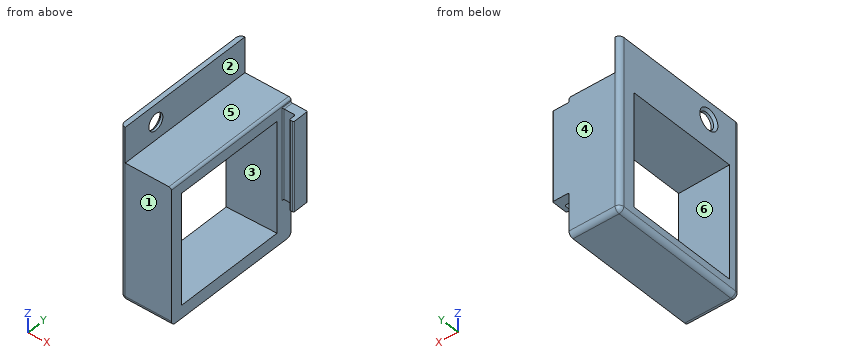
Autodesk Inventor part; units mm, degrees
ref_plane "YZ Plane" through (0, 0, 0) normal (1, 0, 0) x (0, 1, 0)
ref_plane "XZ Plane" through (0, 0, 0) normal (0, 1, 0) x (-1, 0, 0)
ref_plane "XY Plane" through (0, 0, 0) normal (0, 0, 1) x (1, 0, 0)
sketch "Boceto1" plane through (0, 0, 0) normal (1, 0, 0) x (0, 1, 0)
  line L0 (0, 0) -> (-47.8, 0)
  line L1 (-47.8, 0) -> (-47.8, 48)
  line L2 (-47.8, 48) -> (0, 48)
  line L3 (0, 48) -> (0, 0)
  line L4 (-23.9, 48) -> (-23.9, 53)
  line L5 (-23.9, 0) -> (-23.9, -5)
  line L6 (0, 24) -> (5, 24)
  line L7 (-47.8, 24) -> (-52.8, 24)
  line L8 (5, -5) -> (-52.8, -5)
  line L9 (-52.8, -5) -> (-52.8, 53)
  line L10 (-52.8, 53) -> (5, 53)
  line L11 (5, 53) -> (5, -5)
  dimension "d0" = 47.8
  dimension "d1" = 48
  dimension "d2" = 5
  dimension "d3" = 5
  dimension "d4" = 5
  dimension "d5" = 5
extrude "Extrusión1" add sketch "Boceto1" along normal blind 21.5 contours L3 L6 L11 L8 L5 L0 | L5 L8 L9 L7 L1 L0 | L3 L2 L4 L10 L11 L6 | L7 L9 L10 L4 L2 L1
sketch "Boceto2" plane through (0, 0, 0) normal (-1, 0, 0) x (0, 0, 1)
  line L0 (53, 5) -> (53, -52.8)
  line L1 (53, 5) -> (68, 5)
  line L2 (68, 5) -> (68, -52.8)
  line L3 (68, -52.8) -> (53, -52.8)
  line L4 (53, -52.8) -> (53, 5)
  point P0 (0, 0)
  dimension "d8" = 15
extrude "Extrusión2" add sketch "Boceto2" against normal blind 2
sketch "Boceto3" plane through (21.5, 0, 0) normal (1, 0, 0) x (0, 0, -1)
  line L0 (-51, 5) -> (-13, 5)
  line L1 (-13, 3) -> (-51, 3)
  line L2 (-51, 5) -> (-51, 3)
  line L3 (-13, 5) -> (-13, 3)
extrude "Extrusión3" add sketch "Boceto3" along normal blind 7
sketch "Boceto4" plane through (21.5, 3, 13) normal (0, -1, 0) x (1, 0, 0)
  line L0 (0, 38) -> (7, 38)
  line L1 (0, 0) -> (7, 0)
  line L2 (7, 38) -> (5.2, 38)
  line L3 (5.2, 38) -> (5.2, 0)
  line L4 (5.2, 0) -> (7, 0)
  line L5 (7, 0) -> (7, 38)
  point P0 (-21.5, -13)
  point P1 (7, 0)
  dimension "d16" = 1.8
extrude "Extrusión4" add sketch "Boceto4" along normal blind 3
sketch "Boceto5" plane through (0, 0, 0) normal (-1, 0, 0) x (0, 0, 1)
  line L0 (60.5, 5) -> (60.5, -37.5)
  dimension "d19" = 42.5
hole "Agujero1" at (0, -37.5, 60.5) direction (1, 0, 0) diameter 7 depth 2 countersink diameter 9 countersink angle 90
fillet "Empalme3" radius 0.5 2 edges at (28.5, 0, 32) (26.7, 0, 32)
sketch "Boceto6" plane through (21.5, 0, 0) normal (1, 0, 0) x (0, 0, -1)
  line L0 (-48, -47.8) -> (-48, 0)
  line L1 (0, -47.8) -> (-48, -47.8)
  line L2 (-48, 0) -> (-47.5, 0)
  line L3 (-47.5, 0) -> (-47.5, -47.8)
  line L4 (-47.5, -47.8) -> (-48, -47.8)
  line L5 (-48, -47.8) -> (-48, 0)
  line L6 (-48, 0) -> (0, 0)
  line L7 (0, -47.8) -> (-0.5, -47.8)
  line L8 (-0.5, -47.8) -> (-0.5, 0)
  line L9 (-0.5, 0) -> (0, 0)
  line L10 (0, 0) -> (0, -47.8)
  dimension "d30" = 0.5
  dimension "d31" = 0.5
extrude "Extrusión5" add sketch "Boceto6" against normal blind 21.5 contours L0 L2 L3 L1 | L8 L6 L10 L1
chamfer "Chaflán1" distance 0.5 distance2 21.5 2 edges at (0, -23.9, 0.5) (0, -23.9, 47.5) measured on face at (0, -9.3443, 58.8475)
fillet "Empalme4" radius 1 1 edges at (21.5, -23.9, 53)
sketch "Boceto7" plane through (0, 5, -5) normal (0, 1, 0) x (1, 0, 0)
  arc A0 (20.5, -58) -> (21.5, -57) centre (20.5, -57) ccw
  line L0 (21.5, -56) -> (21.5, -57)
  line L1 (21.5, -56) -> (28.5, -56)
  line L2 (28.5, -18) -> (28.5, -56)
  line L3 (21.5, -18) -> (28.5, -18)
  line L4 (21.5, 0) -> (21.5, -18)
  line L5 (0, 0) -> (21.5, 0)
  line L6 (0, 0) -> (0, -73)
  line L7 (0, -73) -> (2, -73)
  line L8 (2, -58) -> (2, -73)
  line L9 (2, -58) -> (20.5, -58)
  point P0 (0, -5)
extrude "Extrusión6" add sketch "Boceto7" along normal blind 2
fillet "Empalme6" radius 2 5 edges at (0, 7, 31.5) (10.75, 7, -5) (0, -22.9, -5) (10.75, -52.8, -5) (0, -52.8, 31.5)
fillet "Empalme7" radius 0.5 5 edges at (28.5, 7, 32) (21.5, 3, 32) (26.7, 3, 32) (21.5, 5, 13) (21.5, 5, 51)
properties part number "cajetinparaestructura"
Check sheet for the modelled part. Datum: model origin and axes. Units: mm. Face numbers are marked on the shaded views. A direction names the side the tool comes from. Give positions to 0.01 mm unless a question says otherwise; leave off trailing zeros. Write each loop counter-clockwise with the first axis right and the second up, starting at its lowest first coordinate (ties: lowest second). Pieces come first, ordered by that corner, then holes. Notation, with made-up numbers: (16, -11) -> (66, -11) arc R9 ccw to (66, -7) -> close; hole circle Ø6 at (-26, 19). An arc over 180 degrees is marked (long way). Use one line per item in the form item = value. Start each with the question number.
1. Access from +Z, -Z, +X, -X, +Y, -Y to the whole of each face (thin tool, end or side, straight path). Record for the marked faces 1 and 2.
2. Section check A-A (z = 6.5). Record the cut outline in (x, y), and give its area (3 significant figures).
3. Mould release check, pull along Y, two halves, no side actions. Record for the marked faces 3, 4, 5 and 6: pulls with the +Y half, pulls with the -Y half, needs draft (parallel to the pull), parting line crosses it, or undercut.
4. Section check C-C (y = -37.5). Count the separate pieces of the cut face and the enclosed holes in it, and give its area (3 significant figures).
5. Section check D-D (x = 3). Record the cut outline in (y, z).
6. Go/stop test with flat-tipped pins: P1, Ø8, axis at y = -36, z = 51.5, coming from the +X side; P2, Ø4.5, axis at y = -14, z = 60, coming from the +X side; P3, Ø0.6, axis at x = 27.5, z = 24, coming from the -Y side. Record where each tip stops, or that it passes through.
7. Thickness scan on line 1 along Y through (x, z) = (1.75, 60.5); line 2 along Y through (x, z) = (6.25, 27); line 3 along Z through (x, y) = (1.4, -37.5). Record the ranges inside material, lowest first. Write a range as from..to.
Conclusion:
q1.face_1 = +Z, -Z, +X, -X, -Y
q1.face_2 = +Z, +X, +Y, -Y
q2.outline = (0, -50.8) arc R2 ccw to (2, -52.8) -> (21.5, -52.8) -> (21.5, -47.8) -> (0, -47.8) -> close; (0, 0) -> (21.5, 0) -> (21.5, 7) -> (2, 7) arc R2 ccw to (0, 5) -> close
q2.area = 256 mm²
q3.face_3 = undercut
q3.face_4 = pulls with the +Y half
q3.face_5 = needs draft
q3.face_6 = undercut
q4.separate_pieces = 3
q4.enclosed_holes = 0
q4.area = 240 mm²
q5.outline = (-52.8, -3) arc R2 ccw to (-50.8, -5) -> (5, -5) arc R2 ccw to (7, -3) -> (7, 53) -> (-52.8, 53) -> close; hole (-47.8, 0.07) -> (0, 0.07) -> (0, 47.93) -> (-47.8, 47.93) -> close
q6.P1 = 21.5
q6.P2 = 2
q6.P3 = 0
q7.line_1 = -52.78..-41, -34..6.98
q7.line_2 = -52.8..-47.8, 0..7
q7.line_3 = -4.91..0.03, 47.97..57, 64..68
